Could you check a few things on this drawing? It's one solid part, dimensions in mm from its lowest x, y, z. A direction names the side the tool comes from. Round coordinates to 2 decimals unless told otherwise and drop trailing zeros. Loops run counter-clockwise (first coordinate to the right, second up) from the corner with the lowest first, then second, coordinate; pieces in that order, holes last. Notation, with made-up numbers: M -17,-24.75 L 35,-24.75 A29 ccw 35,1.25 Z; hole C -28,2.25 d4. An arc over 180 degrees is marked long. Use a Markdown table: item, result. Add a question column.
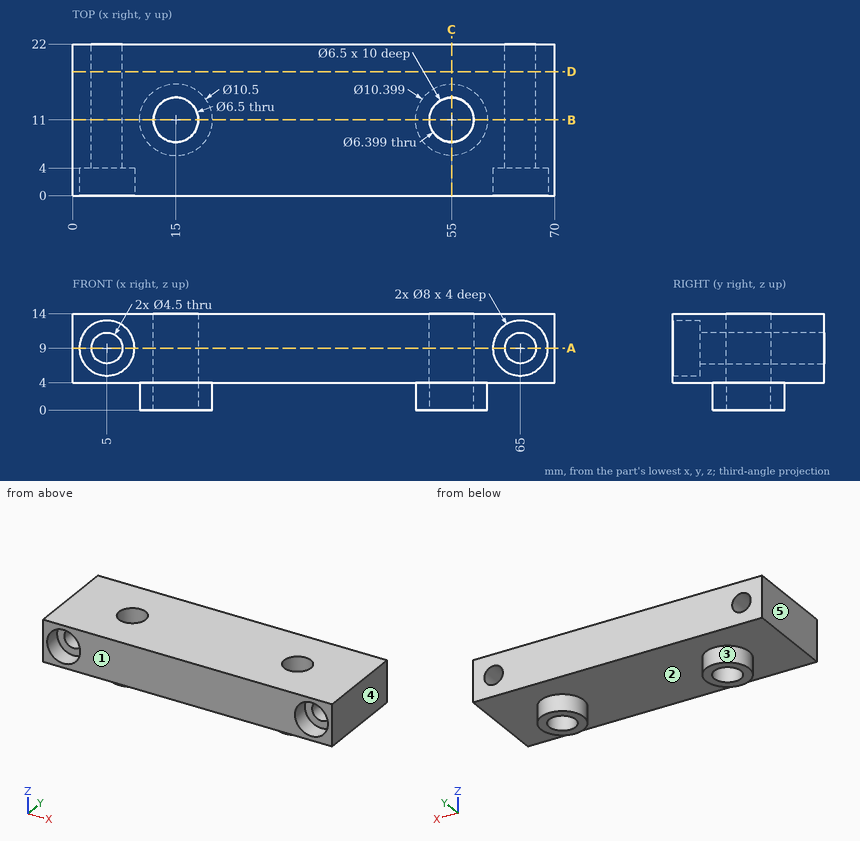
(1) Thinking about a two-plate mould opening in X: for the marked faces 3, 4 and 5, which applies, released by +X, released by -X, zero draft, split by the parting line, or undercut?
(2) Suppose I cut it at C-C on x = 55. List the corners of the cut face in (y, z) for me.
(3) Suppose I cut it at B-B on y = 11. List the corners of the cut face in (x, z) for me.
(4) Suppose I cut it at A-A on z = 9. List the corners of the cut face in (x, y) for me.
(5) If I drill on probe 1 along X at (y, z) = (1.55, 9); probe 2 along X at (y, z) = (4.75, 10.75) (1 decimal); probe 3 along X at (y, z) = (10.5, 9), over which ranges is the centre line in solid material (lowest first)? Write a range as [from, to].
(6) Suppose I cut it at D-D on y = 18. List the corners of the cut face in (x, z) for me, and give its area (3 significant figures).
(7) I'm going to push flat-ended pins straight in: pin 1 (6 mm diameter, centred on x = 65, z = 9, fed in from -Y); pin 2 (11 mm diameter, centred on x = 34, y = 10.5, fed in from -Z); pin 3 (5 mm diameter, centred on x = 15, y = 11, fed in from -Z). Where does each tip first touch, or does it pass through?
(8) On a 3-axis mill with a long thin cutter (end or side, diameter ignored), from which of +Z, -Z, +X, -X, +Y, -Y can I reach the whole of each face in a straight line? I mean the marked faces 1 and 2. Say none if no direction works.
Results below:
| question | item | result |
|---|---|---|
| 1 | face 3 | undercut |
| 1 | face 4 | released by +X |
| 1 | face 5 | released by -X |
| 2 | outline | M 0,4 L 5.8,4 L 5.8,0 L 7.8,0 L 7.8,4 L 7.75,4 L 7.75,14 L 0,14 Z; M 14.2,0 L 16.2,0 L 16.2,4 L 22,4 L 22,14 L 14.25,14 L 14.25,4 L 14.2,4 Z |
| 3 | outline | M 0,4 L 9.75,4 L 9.75,0 L 11.75,0 L 11.75,14 L 0,14 Z; M 18.25,0 L 20.25,0 L 20.25,4 L 49.8,4 L 49.8,0 L 51.8,0 L 51.8,4 L 51.75,4 L 51.75,14 L 18.25,14 Z; M 58.2,0 L 60.2,0 L 60.2,4 L 70,4 L 70,14 L 58.25,14 L 58.25,4 L 58.2,4 Z; hole C 5,9 d4.5; hole C 65,9 d4.5 |
| 4 | outline | M 0,0 L 1,0 L 1,4 L 2.75,4 L 2.75,22 L 0,22 Z; M 7.25,4 L 9,4 L 9,0 L 61,0 L 61,4 L 62.75,4 L 62.75,22 L 7.25,22 Z; M 67.25,4 L 69,4 L 69,0 L 70,0 L 70,22 L 67.25,22 Z; hole C 15,11 d6.5; hole C 55,11 d6.5 |
| 5 | probe 1 | x = [0, 1], [9, 61], [69, 70] |
| 5 | probe 2 | x = [0, 3.6], [6.4, 63.6], [66.4, 70] |
| 5 | probe 3 | x = [0, 2.75], [7.25, 11.79], [18.21, 51.79], [58.21, 62.75], [67.25, 70] |
| 6 | outline | M 0,4 L 70,4 L 70,14 L 0,14 Z; hole C 5,9 d4.5; hole C 65,9 d4.5 |
| 6 | area | 668 mm² |
| 7 | pin 1 | stops at y = 4 |
| 7 | pin 2 | stops at z = 4 |
| 7 | pin 3 | passes through |
| 8 | face 1 | +Z, -Z, +X, -X, -Y |
| 8 | face 2 | -Z |
